Autodesk Inventor part; units mm, degrees
ref_plane "YZ Plane" through (0, 0, 0) normal (1, 0, 0) x (0, 1, 0)
ref_plane "XZ Plane" through (0, 0, 0) normal (0, 1, 0) x (-1, 0, 0)
ref_plane "XY Plane" through (0, 0, 0) normal (0, 0, 1) x (1, 0, 0)
sketch "Esquisse1" plane through (0, 0, 0) normal (0, 0, 1) x (1, 0, 0)
  line L0 (-5, -5) -> (5, -5)
  line L1 (5, -5) -> (5, 5)
  line L2 (5, 5) -> (-5, 5)
  line L3 (-5, 5) -> (-5, -5)
  line L4 (-5, -5) -> (5, 5) construction
  line L5 (5, -5) -> (-5, 5) construction
  arc A0 (5, 5) -> (-5, 5) centre (0, 5) ccw
  point P0 (0, 0)
  dimension "d0" = 10
  dimension "d1" = 10
extrude "Extrusion1" add sketch "Esquisse1" along normal blind 10
hole "Perçage1" at (0, 5, 10) direction (0, 0, -1) diameter 3 end through all
sketch "Esquisse3" plane through (0, 0, 0) normal (1, 0, 0) x (0, 1, 0)
  line L0 (15, 0) -> (15, 10)
  line L1 (3, 0) -> (3, 10)
  line L2 (15, 2.5) -> (3, 2.5)
  line L3 (3, 2.5) -> (3, 7.5)
  line L4 (3, 7.5) -> (15, 7.5)
  line L5 (15, 7.5) -> (15, 2.5)
  line L6 (15, 10) -> (3, 10)
  line L7 (15, 0) -> (3, 0)
  point P0 (0, 0)
  dimension "d23" = 12
  dimension "d29" = 5
  dimension "d30" = 2.5
extrude "Extrusion3" cut sketch "Esquisse3" along normal mid plane 100 contours L2 L1 L4 L0
sketch "Esquisse4" plane through (-5, -5, 0) normal (0, -1, 0) x (1, 0, 0)
  circle A0 centre (5, 5) radius 3
  line L0 (10, 0) -> (10, 10)
  line L1 (0, 10) -> (10, 10)
  line L2 (5, 8) -> (5, 2)
  line L3 (6, 7.8284) -> (6, 2.1716)
  line L4 (4, 7.8284) -> (4, 2.1716)
  line L5 (4, 6.8284) -> (6, 6.8284)
  line L6 (4, 3.1716) -> (6, 3.1716)
  point P0 (5, 0)
  point P1 (5, 6.8284)
  point P2 (4, 5)
  dimension "d24" = 6
  dimension "d25" = 5
  dimension "d26" = 5
  dimension "d37" = 2
  dimension "d38" = 1
  dimension "d39" = 1
  dimension "d40" = 1
  dimension "d41" = 1
extrude "Extrusion4" add sketch "Esquisse4" along normal blind 120
extrude "Extrusion5" cut sketch "Esquisse4" along normal through all contours L3 L5 L2 A0 | A0 L2 L6 L3 | L2 L5 L4 A0 | A0 L4 L6 L2
properties part number "Tige"
Check sheet for the modelled part. Datum: model origin and axes. Units: mm. A direction names the side the tool comes from. Give positions to 0.01 mm unless a question says otherwise; leave off trailing zeros. Write each loop counter-clockwise with the first axis right and the second up, starting at its lowest first coordinate (ties: lowest second). Pieces come first, ordered by that corner, then holes. Notation, with made-up numbers: (67.5, 62) -> (74.5, 62) arc R28 ccw to (74.5, 81) -> close; hole circle Ø3 at (62, -34.5). An arc over 180 degrees is marked (long way). Write item = value, one per line.
Item 1: Scan lines: probe 1 along X at (y, z) = (5, 1.6); probe 2 along Y at (x, z) = (0, 8.65); probe 3 along Z at (x, y) = (-0.75, -49). Record each from-to range of solid material in increasing order. Write a range as from..to.
Output:
probe_1 = -5..-1.5, 1.5..5
probe_2 = -5..3.5, 6.5..10
probe_3 = 3.17..6.83
Item 2: Tool access check on faces 5 (the flat face through (-5, 0, 5)), 6 (the flat face through (0, -5, 3)), 7 (the flat face through (1, 6.5, 7.5)), 8 (the cylindrical face through (0, 10, 1)), 9 (the cylindrical face through (3, -64, 5)). Record the directions out of +Z, -Z, +X, -X, +Y, -Y that give a thin tool (end or side, any length) a straight path to the whole face; none if there is none.
Output:
face_5 = +Z, -Z, -X, +Y, -Y
face_6 = -Y
face_7 = +X, -X, +Y
face_8 = +Z, -Z, +Y
face_9 = +X, -Y
Item 3: Sectioned sample at A-A on y = -44.5. Record the boundary of the cut face in (x, z).
Output:
outline = (-1, 2.17) -> (-1, 3.17) -> (1, 3.17) -> (1, 2.17) arc R3 ccw to (1, 7.83) -> (1, 6.83) -> (-1, 6.83) -> (-1, 7.83) arc R3 ccw to start
Item 4: Gauge pin test, flat ends, axial feed: pin 1 (5 mm diameter, centred on x = 4, z = 7.5, fed in from +Y); pin 2 (0.5 mm diameter, centred on y = -76, z = 2.5, fed in from -X); pin 3 (2.5 mm diameter, centred on x = -1, z = 4.5, fed in from +Y); pin 4 (1.8 mm diameter, centred on x = 0, y = 5, fed in from -Z). Record the tip position at first contact, or that the pin passes through.
Output:
pin_1 = 9.77
pin_2 = -1.98
pin_3 = 3
pin_4 = through
Item 5: Release check for a two-part mould opening along X. For faces 1 (the cylindrical face through (0.9, 6.2, 8.7)), 2 (the flat face through (0, 3, 5)), 3 (the cylindrical face through (0.9, 6.2, 1.2)), 4 (the cylindrical face through (-3, -64, 5)) record: +X half, -X half, draft (parallel to the pull), parting line (faces both ways), or undercut.
Output:
face_1 = undercut
face_2 = draft
face_3 = undercut
face_4 = -X half
Item 6: Sectioned sample at B-B on z = 5. Record the boundary of the cut face in (x, y).
Output:
outline = (-5, -5) -> (-3, -5) -> (-3, -125) -> (3, -125) -> (3, -5) -> (5, -5) -> (5, 3) -> (-5, 3) -> close
